from build123d import *

# Parameters (mm, degrees)
EXTRUDE_2_DEPTH     = 20
CUT_EXTRUDE_1_REACH = 76.191
SKETCH_3_W          = 14
SKETCH_3_H          = 20
SKETCH_4_R          = 2
CUT_EXTRUDE_2_DEPTH = 10
SKETCH_5_R          = 1.5
CUT_EXTRUDE_3_DEPTH = 10


with BuildPart() as part:
    # Эскиз2 → Бобышка-Вытянуть2 (new body)
    with BuildSketch(Plane.XY):
        Polygon((0, 0), (60.5, 0), (60.5, 38), (50.5, 38), (50.5, 3), (10, 3), (10, 38), (0, 38), align=None)
    extrude(amount=EXTRUDE_2_DEPTH)

    # Эскиз3 → Вырез-Вытянуть1 (cut, up to next)
    with BuildSketch(Plane.ZY, mode=Mode.PRIVATE) as cut_extrude_1_sk1:
        with Locations((10, 13)):
            Rectangle(SKETCH_3_W, SKETCH_3_H)
    cut_extrude_1_tool1 = extrude(cut_extrude_1_sk1.sketch, amount=-CUT_EXTRUDE_1_REACH, mode=Mode.PRIVATE) & part.part
    add(cut_extrude_1_tool1.solids().sort_by_distance((0, 13, 10))[0], mode=Mode.SUBTRACT)

    # Эскиз4 → Вырез-Вытянуть2 (cut)
    with BuildSketch(Plane(origin=(0, 38, 0), x_dir=(1, 0, 0), z_dir=(0, 1, 0))):
        with Locations(Location((5, -5, 0), (0, 0, 270))):
            Circle(SKETCH_4_R)
        with Locations(Location((5, -15, 0), (0, 0, 270))):
            Circle(SKETCH_4_R)
        with Locations(Location((55.5, -5, 0), (0, 0, 270))):
            Circle(SKETCH_4_R)
        with Locations(Location((55.5, -15, 0), (0, 0, 270))):
            Circle(SKETCH_4_R)
    extrude(amount=-CUT_EXTRUDE_2_DEPTH, mode=Mode.SUBTRACT)

    # Эскиз5 → Вырез-Вытянуть3 (cut)
    with BuildSketch(Plane.XZ):
        with Locations(Location((20, 10, 0), (0, 0, 270))):
            Circle(SKETCH_5_R)
        with Locations(Location((40.5, 10, 0), (0, 0, 270))):
            Circle(SKETCH_5_R)
    extrude(amount=-CUT_EXTRUDE_3_DEPTH, mode=Mode.SUBTRACT)


solid = part.part
Verification items for the finished model (mm, model axes). A direction names the side the tool comes from. Give positions to 0.01 mm unless a question says otherwise; leave off trailing zeros. Loops run counter-clockwise (first coordinate to the right, second up) from the corner with the lowest first, then second, coordinate; pieces in that order, holes last.
1) Set-up check for faces 5 (the flat face through (50.5, 21, 10)), 6 (the flat face through (25, 3, 10)), 7 (the flat face through (5, 28, 5)): record each of +Z, -Z, +X, -X, +Y, -Y from which the full face is reachable in a straight line by a thin tool's end or side.
2) Sectioned sample at C-C, the plane y = 32. Enter the section's corners in (x, z).
3) Thickness scan on line 1 along X through (y, z) = (0.8, 10); line 2 along X through (y, z) = (31.75, 15); line 3 along X through (y, z) = (34.5, 15.5). Record the ranges inside material, lowest first.
4) Sectioned sample at A-A, the plane y = 16.5. Enter the section's corners in (x, z), then the cut area to 3 significant figures.
5) Draft check along Z on faces 1 (the cylindrical face through (57.483, 33.07, 4.74)), 2 (the cylindrical face through (5, 33, 3)), 3 (the flat face through (23, 2, 0)), 4 (the flat face through (30, 0, 10)). Enter one of: pulls with the +Z half, pulls with the -Z half, needs draft (parallel to the pull), parting line crosses it, or undercut.
6) Sectioned sample at D-D, the plane z = 5. Enter the section's corners in (x, y), then the cut area to 4 significant figures.
7) Sectioned sample at B-B, the plane x = 20. Enter the section's corners in (y, z).
8) Depth check by flat-ended pin: pin 1 Ø4.5 at (x, z) = (5, 5) entering from -Y; pin 2 Ø2.5 at (x, z) = (20, 10) entering from -Y; pin 3 Ø6 at (x, z) = (26.5, 7.5) entering from +Y; pin 4 Ø1.2 at (x, z) = (5, 5.5) entering from +Y. Enter the tip coordinate at first touch or a pass-through.
Answers:
1. face 5: +Z, -Z, +Y
1. face 6: none
1. face 7: +Y
2. outline: (0, 0) - (10, 0) - (10, 20) - (0, 20) - close; (50.5, 0) - (60.5, 0) - (60.5, 20) - (50.5, 20) - close; hole circle Ø4 at (5, 5); hole circle Ø4 at (5, 15); hole circle Ø4 at (55.5, 5); hole circle Ø4 at (55.5, 15)
3. line 1: x = 0 to 18.5, 21.5 to 39, 42 to 60.5
3. line 2: x = 0 to 3, 7 to 10, 50.5 to 53.5, 57.5 to 60.5
3. line 3: x = 0 to 3.06, 6.94 to 10, 50.5 to 53.56, 57.44 to 60.5
4. outline: (0, 0) - (10, 0) - (10, 3) - (0, 3) - close; (0, 17) - (10, 17) - (10, 20) - (0, 20) - close; (50.5, 0) - (60.5, 0) - (60.5, 20) - (50.5, 20) - close
4. area: 260 mm2
5. face 1: undercut
5. face 2: undercut
5. face 3: pulls with the -Z half
5. face 4: needs draft
6. outline: (0, 0) - (60.5, 0) - (60.5, 38) - (57.5, 38) - (57.5, 28) - (53.5, 28) - (53.5, 38) - (50.5, 38) - (50.5, 3) - (0, 3) - close; (0, 23) - (10, 23) - (10, 38) - (7, 38) - (7, 28) - (3, 28) - (3, 38) - (0, 38) - close
6. area: 601.5 mm2
7. outline: (0, 0) - (3, 0) - (3, 8.5) - (0, 8.5) - close; (0, 11.5) - (3, 11.5) - (3, 20) - (0, 20) - close
8. pin 1: stops at y = 0
8. pin 2: passes through
8. pin 3: stops at y = 3
8. pin 4: stops at y = 28
